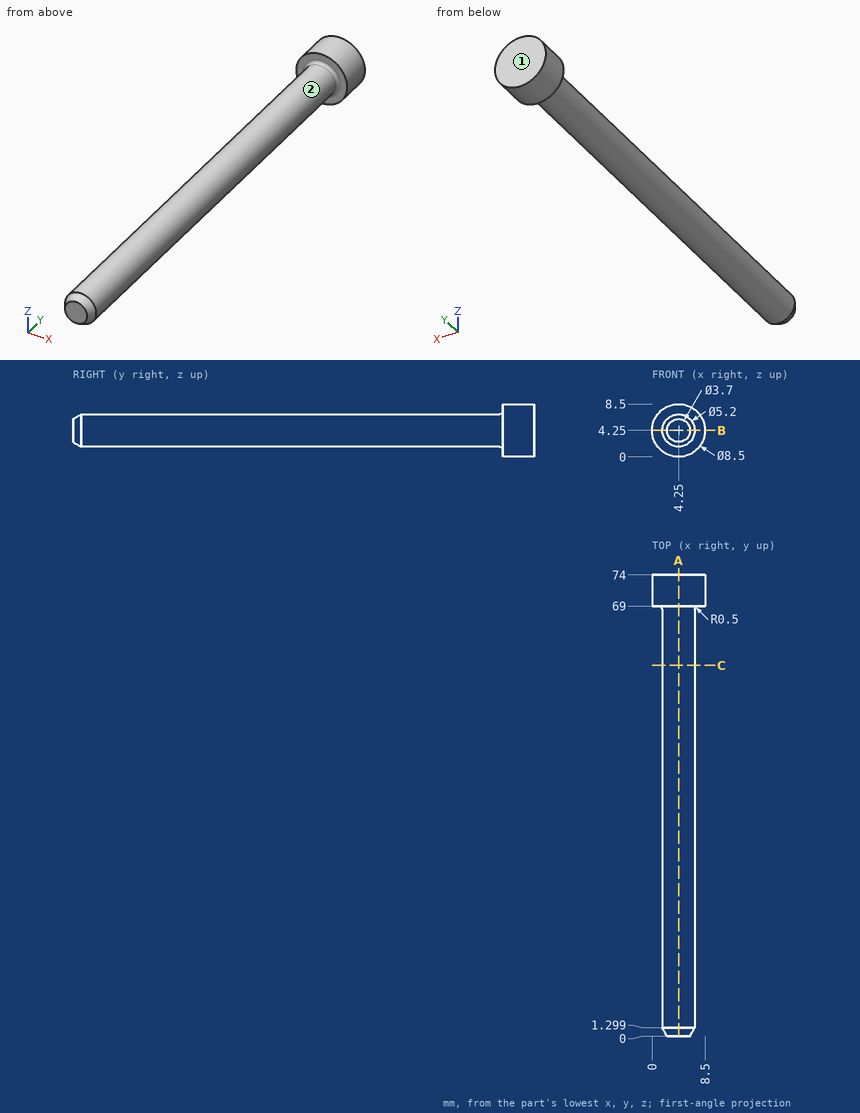
Geometry: see drawing. Coordinates: mm, zero at the bounding-box minimum. A direction names the side the tool comes from. Coordinates: 2 decimals unless noted, no trailing zeros. Loops run counter-clockwise (first coordinate to the right, second up) from the corner with the lowest first, then second, coordinate; pieces in that order, holes last. Notation, with made-up numbers: M 24,-36.5 L 41,-36.5 A19 ccw 41,-8.5 Z; hole C 73,86 d10. An arc over 180 degrees is marked long. Put each result on its own line as item: value. Start each with the question number.
1) Contact query for flat-ended pins moving along their axis: pin 1 Ø2 at (y, z) = (54.5, 4) entering from -X; pin 2 Ø2 at (y, z) = (31.5, 7) entering from +X; pin 3 Ø4 at (x, y) = (1, 26) entering from -Z. Output: stop coordinate, or through.
2) Cut plane A-A on x = 4.25. Return the cut outline in (y, z), then the cut area to 3 significant figures.
3) Ray query, L1, parallel to Y at x = 1.25, z = 4; L2, parallel to Z at x = 2.25, y = 58; L3, parallel to X at y = 42, z = 3.25. Return the intervals inside material, ascending. Write a range as from..to.
4) Cut plane C-C on y = 59.5. Return the cut outline in (x, z).
5) Cut plane B-B on z = 4.25. Return the cut outline in (x, y).
6) Reachability of the marked faces 1 and 2 from +Z, -Z, +X, -X, +Y, -Y: full face, straight path, thin tool, end or side. Return the list, or none.
The answers:
1. pin 1: stops at x = 1.65
1. pin 2: stops at x = 6.17
1. pin 3: stops at z = 1.97
2. outline: M 0,2.4 L 1.3,1.65 L 68.5,1.65 A0.5 cw 69,1.15 L 69,0 L 74,0 L 74,8.5 L 69,8.5 L 69,7.35 A0.5 cw 68.5,6.85 L 1.3,6.85 L 0,6.1 Z
2. area: 400 mm²
3. L1: y = 68.99..74
3. L2: z = 2.59..5.91
3. L3: x = 1.85..6.65
4. outline: C 4.25,4.25 d5.2
5. outline: M 0,69 L 1.15,69 A0.5 cw 1.65,68.5 L 1.65,1.3 L 2.4,0 L 6.1,0 L 6.85,1.3 L 6.85,68.5 A0.5 cw 7.35,69 L 8.5,69 L 8.5,74 L 0,74 Z
6. face 1: +Z, -Z, +X, -X, +Y
6. face 2: -Y
